Can you work these out from the model? Positions are in its coordinate system, mm. A direction names the side the tool comes from. Coordinates: 2 decimals unless noted, no trailing zeros. Order: outer loops, then holes, each group sorted by start corner. A loop starts at its lowest first (then second) coordinate and runs counter-clockwise, first axis right, second up. Notation, with made-up numbers: (53, 3.5) -> (96, 3.5) arc R15 ccw to (96, 13.5) -> close; hole circle Ø10 at (-36, 32.5). An arc over 180 degrees is marked (long way). Answer as a JSON object with one key per item and string values. Group by question number.
(1) If we mould it in two halves opening along Y, with no side actions, what happens to faces 1 (the flat face through (296, 0, 49)), 2 (the flat face through (296, -419, 0)), 3 (the flat face through (296, -12, 55)), 4 (the flat face through (299, -875, 40))? For each: pulls with the +Y half, pulls with the -Y half, needs draft (parallel to the pull), parting line crosses it, or undercut.
(2) Which directions (+Z, -Z, +X, -X, +Y, -Y) give clear straight access to the entire face, cutting with the end or side of a thin tool? Please do faces 5 (the flat face through (375, -862, 40)), 6 (the flat face through (225, -862, 40)), 7 (the flat face through (299, -862, 50)), 8 (the flat face through (296, -419, 12)), 9 (the flat face through (299, -862, 30)).
(3) I want a section at C-C, the plane x = 452.5. List the corners of the cut face in (y, z) for me.
(4) For pin 1 (12.5 mm diameter, centred on x = 334.5, y = -861, fed in from -Z); pin 2 (4 mm diameter, centred on x = 80.5, z = 30, fed in from -Y); pin 3 (12.5 mm diameter, centred on x = 274.5, y = -867.5, fed in from +Z), each with a flat end and sliding along its axis, tell me the tip position at first contact or that it passes through.
(5) I want a section at B-B, the plane y = -78. List the corners of the cut face in (x, z) for me.
(6) I need wall thicknesses on line 1 (Y direction, x = 39.5, z = 78); line 2 (X direction, y = -263, z = 66); line 3 (Y direction, x = 245.5, z = 47). Which ranges of each line are inside material? Lowest first, please.
(7) I want a section at A-A, the plane z = 62. List the corners of the cut face in (x, y) for me, plus the area to 3 significant figures.
from build123d import *

# Parameters (mm, degrees)
F0_W     = 600
F0_H     = 850
F1_DEPTH = 12
F2_W     = 600
F2_H     = 850
F2_W_2   = 576
F2_H_2   = 826
F3_DEPTH = 88
F4_W     = 150
F4_H     = 20
F5_DEPTH = 25


with BuildPart() as f1:
    # F0 (on Top) → F1 (new body)
    with BuildSketch(Plane.XY):
        with Locations((300, -425)):
            Rectangle(F0_W, F0_H)
    extrude(amount=F1_DEPTH)

    # F2 (on face) → F3 (join)
    with BuildSketch(Plane.XY.offset(12)):
        with Locations((300, -425)):
            Rectangle(F2_W, F2_H)
        with Locations((300, -425)):
            Rectangle(F2_W_2, F2_H_2, mode=Mode.SUBTRACT)
    extrude(amount=F3_DEPTH)

    # F4 (on face) → F5 (join)
    with BuildSketch(Plane.XZ.offset(850)):
        with Locations((300, 40)):
            Rectangle(F4_W, F4_H)
    extrude(amount=F5_DEPTH)


solid = f1.part
Computed values:
{
 "1": {"face 1": "pulls with the +Y half", "face 2": "needs draft", "face 3": "undercut", "face 4": "pulls with the -Y half"},
 "2": {"face 5": "+Z, -Z, +X, -Y", "face 6": "+Z, -Z, -X, -Y", "face 7": "+Z, +X, -X, -Y", "face 8": "+Z", "face 9": "-Z, +X, -X, -Y"},
 "3": {"outline": "(-850, 0) -> (0, 0) -> (0, 100) -> (-12, 100) -> (-12, 12) -> (-838, 12) -> (-838, 100) -> (-850, 100) -> close"},
 "4": {"pin 1": "stops at z = 30", "pin 2": "stops at y = -850", "pin 3": "stops at z = 50"},
 "5": {"outline": "(0, 0) -> (600, 0) -> (600, 100) -> (588, 100) -> (588, 12) -> (12, 12) -> (12, 100) -> (0, 100) -> close"},
 "6": {"line 1": "y = -850 to -838, -12 to 0", "line 2": "x = 0 to 12, 588 to 600", "line 3": "y = -875 to -838, -12 to 0"},
 "7": {"outline": "(0, -850) -> (600, -850) -> (600, 0) -> (0, 0) -> close; hole (12, -838) -> (588, -838) -> (588, -12) -> (12, -12) -> close", "area": "34,200 mm2"}
}
